For this review, take the finished solid that the model builds, in its own axes (mm). Face numbers are marked on the shaded views. Give positions to 0.01 mm unless a question says otherwise; leave off trailing zeros. Write each loop counter-clockwise with the first axis right and the second up, starting at its lowest first coordinate (ties: lowest second). Pieces come first, ordered by that corner, then holes. Notation, with made-up numbers: M 63.25,-12 L 112.25,-12 A20 ccw 112.25,18 Z; hole C -27.75,5.25 d6. An arc over 180 degrees is marked long. Answer as a JSON object with one key per item and string values. Group by question number.
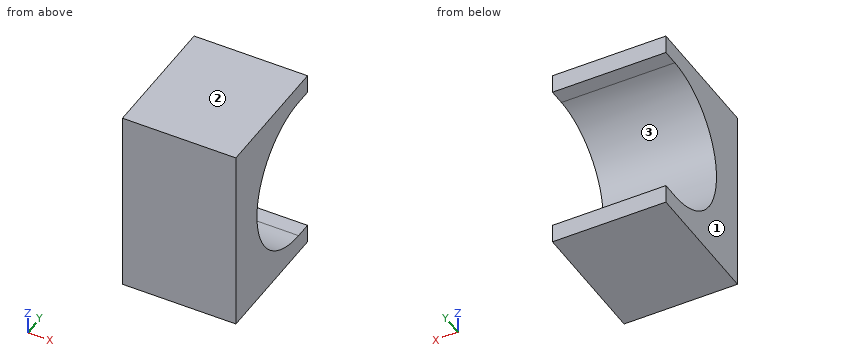
```python
from build123d import *

# Parameters (mm, degrees)
SKETCH1_W           = 35
SKETCH1_H           = 58
BOSS_EXTRUDE1_DEPTH = 40
CUT_EXTRUDE1_DEPTH  = 61.547502013


with BuildPart() as part:
    # Sketch1 → Boss-Extrude1 (new body)
    with BuildSketch(Plane(origin=(0, 0, 0), x_dir=(1, 0, 0), z_dir=(0, 1, 0))):
        Rectangle(SKETCH1_W, SKETCH1_H)
    extrude(amount=BOSS_EXTRUDE1_DEPTH)

    # Sketch2 → Cut-Extrude1 (cut, through all)
    with BuildSketch(Plane(origin=(17.5, 0, 0), x_dir=(0, 0, -1), z_dir=(1, 0, 0))):
        with BuildLine():
            Line((-23.25, 35), (-23.25, 58.25))
            Line((-23.25, 58.25), (23.25, 58.25))
            Line((23.25, 58.25), (23.25, 35))
            ThreePointArc((23.25, 35), (0, 11.75), (-23.25, 35))
        make_face()
    extrude(amount=-CUT_EXTRUDE1_DEPTH, mode=Mode.SUBTRACT)


solid = part.part
```
Item 1: To check wall thickness, follow probe 1 along Z at (x, y) = (13, 37.5); probe 2 along Z at (x, y) = (-10.5, 20); probe 3 along Y at (x, z) = (12.5, 12). State the ranges of each line that lie inside material, in increasing order.
Item 2: Consider section B-B (x = 9). Give the boundary of the cut face in (y, z), plus the area to 3 significant figures.
Item 3: Consider section D-D (z = 0). Give the boundary of the cut face in (x, y).
Item 4: Consider section A-A (y = 13). Give the boundary of the cut face in (x, z).
Item 5: Insertion check: P1, Ø6, axis at x = -11.5, z = -15, coming from the +Y side; P2, Ø12, axis at x = -2.5, z = 7, coming from the +Y side; P3, Ø8, axis at x = 0, z = -15.5, coming from the +Y side. Each pin has a flat end and moves straight along its axis. Give the tip position at first contact, or say it passes through.
Item 6: Consider section C-C (y = 33). Give the boundary of the cut face in (x, z).
Item 7: Draft analysis for pull direction Z (two halves, no side actions). For the marked faces 1, 2 and 3, state which applies: released by +Z, released by -Z, zero draft, split by the parting line, or undercut.
Result set:
{
 "1": {"probe 1": "z = -29 to -23.25, 23.25 to 29", "probe 2": "z = -29 to -17.76, 17.76 to 29", "probe 3": "y = 0 to 15.09"},
 "2": {"outline": "M 0,-29 L 40,-29 L 40,-23.25 L 35,-23.25 A23.25 cw 35,23.25 L 40,23.25 L 40,29 L 0,29 Z", "area": "1,240 mm^2"},
 "3": {"outline": "M -17.5,0 L 17.5,0 L 17.5,11.75 L -17.5,11.75 Z"},
 "4": {"outline": "M -17.5,-29 L 17.5,-29 L 17.5,-7.52 L -17.5,-7.52 Z; M -17.5,7.52 L 17.5,7.52 L 17.5,29 L -17.5,29 Z"},
 "5": {"P1": "stops at y = 20.28", "P2": "stops at y = 15.72", "P3": "stops at y = 22.34"},
 "6": {"outline": "M -17.5,-29 L 17.5,-29 L 17.5,-23.16 L -17.5,-23.16 Z; M -17.5,23.16 L 17.5,23.16 L 17.5,29 L -17.5,29 Z"},
 "7": {"face 1": "zero draft", "face 2": "released by +Z", "face 3": "undercut"}
}
